from build123d import *

# Parameters (mm, degrees)
CUT_EXTRUDE1_DEPTH = 4
CHAMFER1_SIZE      = 1


with BuildPart() as part:
    # Sketch1 → Revolve1 (revolve)
    with BuildSketch(Plane.XY):
        Polygon((0, 0), (0, 8), (3, 8), (3, 6), (173.8, 6), (173.8, 0), align=None)
    revolve(axis=Axis((173.8, 0, 0), (-1, 0, 0)))

    # Sketch2 → Cut-Extrude1 (cut)
    with BuildSketch(Plane.ZY):
        Polygon((0, 5), (-4.330127019, 2.5), (-4.330127019, -2.5), (0, -5), (4.330127019, -2.5), (4.330127019, 2.5), align=None)
    extrude(amount=-CUT_EXTRUDE1_DEPTH, mode=Mode.SUBTRACT)

    # Chamfer1
    chamfer1_edges = [part.edges().sort_by_distance(p)[0] for p in [
        (173.8, -6, 0),
        (0, -8, 0),
    ]]
    chamfer(chamfer1_edges, length=CHAMFER1_SIZE)


solid = part.part
Part model, mm, in its own coordinate system. A direction names the side the tool comes from. Coordinates: 2 decimals unless noted, no trailing zeros. Loops run counter-clockwise (first coordinate to the right, second up) from the corner with the lowest first, then second, coordinate; pieces in that order, holes last. Notation, with made-up numbers: M -1,1.25 L 14,1.25 A10 ccw 14,12.25 Z; hole C 44,-10 d3. An arc over 180 degrees is marked long. Use a Markdown table: item, result. Add a question column.
Q1. Which spindle directions (+Z, -Z, +X, -X, +Y, -Y) get a long thin tool onto all of the face, cutting with end or side? Do faces 5 (the cylindrical face through (89, -6, 0)), 6 (the flat face through (1.97, 3.73, 2.2)), 7 (the flat face through (173.8, 0, 0)). Say none if no direction does.
Q2. Probe L1, parallel to X at y = 6.25, z = -1.25; L2, parallel to Z at x = 68.5, y = -0.25; L3, parallel to Y at x = 43, z = -0.5. List the from-to ranges inside material, lowest first.
Q3. Pin check, flat tips, straight feed: P1, Ø8, axis at x = 56.5, y = -1, coming from the +Z side; P2, Ø2, axis at x = 143.5, y = 6, coming from the +Z side; P3, Ø6, axis at x = 94, z = -2, coming from the -Y side. Stop position of each tip, or through.
Q4. Cut at A-A (y = 0). Write the cut outline in (x, z), and give its area (3 significant figures).
Q5. Mould opens along Z. For faces 1 (the cylindrical face through (2.01, -1.73, 7.81)), 2 (the flat face through (3, -2, -6)), 3 (the flat face through (1.97, 3.77, -2.13)), 4 (the flat face through (2, 0, -4.33)) say: +Z half, -Z half, draft (parallel to the pull), parting line (faces both ways), or undercut.
Q6. Cut at B-B (x = 100). Write the cut outline in (y, z).
Worked out:
| question | item | result |
|---|---|---|
| 1 | face 5 | +X |
| 1 | face 6 | -X |
| 1 | face 7 | +Z, -Z, +X, +Y, -Y |
| 2 | L1 | x = 0 to 3 |
| 2 | L2 | z = -5.99 to 5.99 |
| 2 | L3 | y = -5.98 to 5.98 |
| 3 | P1 | stops at z = 6 |
| 3 | P2 | stops at z = 3.32 |
| 3 | P3 | stops at y = -6 |
| 4 | outline | M 0,-7 L 1,-8 L 3,-8 L 3,-6 L 172.8,-6 L 173.8,-5 L 173.8,5 L 172.8,6 L 3,6 L 3,8 L 1,8 L 0,7 L 0,4.33 L 4,4.33 L 4,-4.33 L 0,-4.33 Z |
| 4 | area | 2,060 mm2 |
| 5 | face 1 | parting line |
| 5 | face 2 | draft |
| 5 | face 3 | undercut |
| 5 | face 4 | undercut |
| 6 | outline | C 0,0 d12 |
